```python
from build123d import *

# Parameters (mm, degrees)
BOSS_EXTRUDE1_DEPTH     = 3
BOSS_EXTRUDE2_DEPTH     = 12
BOSS_EXTRUDE3_DEPTH     = 4.17
CUT_EXTRUDE1_DEPTH      = 100.227239708
CUT_EXTRUDE1_DEPTH_BACK = 100.227239708
SKETCH3_R               = 2
CHAMFER1_SIZE           = 10
SKETCH8_R               = 4
CUT_EXTRUDE2_DEPTH      = 16.17
CHAMFER2_SIZE           = 1


with BuildPart() as part:
    # Sketch1 → Boss-Extrude1 (new body)
    with BuildSketch(Plane(origin=(0, 0, 0), x_dir=(1, 0, 0), z_dir=(0, 1, 0))):
        Polygon((-94.41, 0), (94.41, 0), (68.5, 25.91), (-68.5, 25.91), align=None)
    extrude(amount=BOSS_EXTRUDE1_DEPTH)

    # Sketch5 → Boss-Extrude2 (add)
    with BuildSketch(Plane(origin=(0, 3, 0), x_dir=(1, 0, 0), z_dir=(0, 1, 0))):
        with BuildLine():
            Line((-64.496944889, 25.91), (-68.5, 25.91))
            Line((-68.5, 25.91), (-94.41, 0))
            Line((-94.41, 0), (94.41, 0))
            Line((94.41, 0), (68.5, 25.91))
            Line((68.5, 25.91), (64.496944889, 25.91))
            ThreePointArc((64.496944889, 25.91), (54.829686624, 24.966540009), (45.527255216, 22.171764706))
            ThreePointArc((45.527255216, 22.171764706), (0, 13.2), (-45.527255216, 22.171764706))
            ThreePointArc((-45.527255216, 22.171764706), (-54.829686624, 24.966540009), (-64.496944889, 25.91))
        make_face()
    extrude(amount=BOSS_EXTRUDE2_DEPTH)

    # Sketch7 → Boss-Extrude3 (add)
    with BuildSketch(Plane(origin=(0, 15, 0), x_dir=(1, 0, 0), z_dir=(0, 1, 0))):
        Polygon((-94.41, 0), (-68.5, 25.91), (68.5, 25.91), (94.41, 0), align=None)
    extrude(amount=BOSS_EXTRUDE3_DEPTH)

    # Sketch3 → Cut-Extrude1 (cut, two sides: drawn at the far end of the back side and taken through both)
    with BuildSketch(Plane(origin=(0, 3, 0), x_dir=(1, 0, 0), z_dir=(0, 1, 0)).offset(-CUT_EXTRUDE1_DEPTH_BACK)):
        with Locations(Location((-35.355339059, 12.955, 0), (0, 0, 270))):
            Circle(SKETCH3_R)
        with Locations(Location((35.355339059, 12.955, 0), (0, 0, 270))):
            Circle(SKETCH3_R)
    extrude(amount=CUT_EXTRUDE1_DEPTH + CUT_EXTRUDE1_DEPTH_BACK, mode=Mode.SUBTRACT)

    # Chamfer1
    chamfer1_edges = [part.edges().sort_by_distance(p)[0] for p in [
        (0, 19.17, 0),
    ]]
    chamfer(chamfer1_edges, length=CHAMFER1_SIZE)

    # Sketch8 → Cut-Extrude2 (cut)
    with BuildSketch(Plane(origin=(0, 19.17, 0), x_dir=(1, 0, 0), z_dir=(0, 1, 0))):
        with Locations(Location((-35.355339059, 12.955, 0), (0, 0, 270))):
            Circle(SKETCH8_R)
        with Locations(Location((35.355339059, 12.955, 0), (0, 0, 270))):
            Circle(SKETCH8_R)
    extrude(amount=-CUT_EXTRUDE2_DEPTH, mode=Mode.SUBTRACT)

    # Chamfer2
    chamfer2_edges = [part.edges().sort_by_distance(p)[0] for p in [
        (-35.355339059, 19.17, -16.955),
        (35.355339059, 19.17, -16.955),
    ]]
    chamfer(chamfer2_edges, length=CHAMFER2_SIZE)


solid = part.part
```
Geometry check sheet. Reference: the model listing, model coordinates, mm. A direction names the side the tool comes from. Give positions to 0.01 mm unless a question says otherwise; leave off trailing zeros. Write each loop counter-clockwise with the first axis right and the second up, starting at its lowest first coordinate (ties: lowest second). Pieces come first, ordered by that corner, then holes. Notation, with made-up numbers: (-8, 43) - (30, 43) arc R14 cw to (30, 54) - close; hole circle Ø7 at (-32.75, 39). An arc over 180 degrees is marked (long way). Use a Markdown table: item, result.
Q1. Go/stop test with flat-tipped pins: P1, Ø6.5, axis at x = -35.36, z = -12.96, coming from the +Y side; P2, Ø8, axis at y = 2, z = -8.5, coming from the +X side; P3, Ø2, axis at x = 17.5, y = 13.5, coming from the +Z side. Record where each tip stops, or that it passes through.
Computed:
| item | result |
|---|---|
| P1 | stops at y = 3 |
| P2 | stops at x = 89.91 |
| P3 | stops at z = -3.33 |
Q2. Section check A-A, the plane x = -79. Enter the section's corners in (y, z).
Computed:
| item | result |
|---|---|
| outline | (0, -15.41) - (19.17, -15.41) - (19.17, -10) - (9.17, 0) - (0, 0) - close |
Q3. Section check B-B, the plane z = -5.5. Enter the section's corners in (x, y), then the cut area to 3 significant figures.
Computed:
| item | result |
|---|---|
| outline | (-88.91, 0) - (88.91, 0) - (88.91, 14.67) - (-88.91, 14.67) - close |
| area | 2,610 mm² |
Q4. Set-up check for faces 1 (the face through (-31.39, 10.69, -13.48)), 2 (the face through (1, 5, 0)), 3 (the face through (1, 15, -21)): record each of +Z, -Z, +X, -X, +Y, -Y from which the full face is reachable in a straight line by a thin tool's end or side.
Computed:
| item | result |
|---|---|
| face 1 | +Y |
| face 2 | +Z, +X, -X, +Y, -Y |
| face 3 | -Z |
Q5. Section check C-C, the plane x = 16.5. Enter the section's corners in (y, z), then the cut area to 3 significant figures.
Computed:
| item | result |
|---|---|
| outline | (0, -25.91) - (3, -25.91) - (3, -14.34) - (15, -14.34) - (15, -25.91) - (19.17, -25.91) - (19.17, -10) - (9.17, 0) - (0, 0) - close |
| area | 308 mm² |
Q6. Thickness scan on L1, parallel to Y at x = 28.5, z = -21; L2, parallel to X at y = 9, z = -11.25; L3, parallel to X at y = 9.25, z = -12.25. Record the ranges inside material, lowest first. Write a range as [from, to].
Computed:
| item | result |
|---|---|
| L1 | y = [0, 3], [15, 19.17] |
| L2 | x = [-83.16, -38.97], [-31.74, 31.74], [38.97, 83.16] |
| L3 | x = [-82.16, -39.29], [-31.42, 31.42], [39.29, 82.16] |
Q7. Section check D-D, the plane x = 81.5. Enter the section's corners in (y, z).
Computed:
| item | result |
|---|---|
| outline | (0, -12.91) - (19.17, -12.91) - (19.17, -10) - (9.17, 0) - (0, 0) - close |
Q8. Draft check along X on faces 4 (the face through (-1, 0, -13)), 5 (the face through (55, 9, -25)), 6 (the face through (-55, 9, -25)), 7 (the face through (81.27, 9.45, -13.14)). Enter one of: pulls with the +X half, pulls with the -X half, needs draft (parallel to the pull), parting line crosses it, or undercut.
Computed:
| item | result |
|---|---|
| face 4 | needs draft |
| face 5 | undercut |
| face 6 | undercut |
| face 7 | pulls with the +X half |
